```python
from build123d import *

# Parameters (mm, degrees)
SKETCH1_W           = 92
SKETCH1_H           = 56
BOSS_EXTRUDE1_DEPTH = 12
SKETCH8_W           = 92
SKETCH8_H           = 2
BOSS_EXTRUDE3_DEPTH = 12
CUT_EXTRUDE1_REACH  = 58.214
SKETCH2_R           = 10.5
CUT_EXTRUDE5_REACH  = 58.214
FILLET2_R           = 12
CUT_EXTRUDE6_DEPTH  = 6
CUT_EXTRUDE7_REACH  = 58.214
SKETCH12_R          = 2.25
SKETCH12_R_2        = 10.5


with BuildPart() as part:
    # Sketch1 → Boss-Extrude1 (new body)
    with BuildSketch(Plane(origin=(0, 0, 0), x_dir=(1, 0, 0), z_dir=(0, 1, 0))):
        Rectangle(SKETCH1_W, SKETCH1_H)
    extrude(amount=BOSS_EXTRUDE1_DEPTH)

    # Sketch8 → Boss-Extrude3 (add)
    with BuildSketch(Plane(origin=(0, 12, 0), x_dir=(1, 0, 0), z_dir=(0, 1, 0))):
        with Locations((0, 29)):
            Rectangle(SKETCH8_W, SKETCH8_H)
    extrude(amount=-BOSS_EXTRUDE3_DEPTH)

    # Sketch2 → Cut-Extrude1 (cut, up to next)
    with BuildSketch(Plane(origin=(0, 12, 0), x_dir=(1, 0, 0), z_dir=(0, 1, 0)), mode=Mode.PRIVATE) as cut_extrude1_sk1:
        with Locations(Location((-25, -1.5, 0), (0, 0, 270))):
            Circle(SKETCH2_R)
    cut_extrude1_tool1 = extrude(cut_extrude1_sk1.sketch, amount=-CUT_EXTRUDE1_REACH, mode=Mode.PRIVATE) & part.part
    # Sketch2 → Cut-Extrude1 (cut, up to next)
    with BuildSketch(Plane(origin=(0, 12, 0), x_dir=(1, 0, 0), z_dir=(0, 1, 0)), mode=Mode.PRIVATE) as cut_extrude1_sk2:
        with Locations(Location((25, -1.5, 0), (0, 0, 270))):
            Circle(SKETCH2_R)
    cut_extrude1_tool2 = extrude(cut_extrude1_sk2.sketch, amount=-CUT_EXTRUDE1_REACH, mode=Mode.PRIVATE) & part.part
    add(cut_extrude1_tool1.solids().sort_by_distance((-25, 12, 1.5))[0], mode=Mode.SUBTRACT)
    add(cut_extrude1_tool2.solids().sort_by_distance((25, 12, 1.5))[0], mode=Mode.SUBTRACT)

    # Sketch10 → Cut-Extrude5 (cut, up to next)
    with BuildSketch(Plane(origin=(0, 12, 0), x_dir=(1, 0, 0), z_dir=(0, 1, 0)), mode=Mode.PRIVATE) as cut_extrude5_sk1:
        with BuildLine():
            Line((-46, 5.057438524), (-46, 30))
            Line((-46, 30), (-16, 30))
            Line((-16, 30), (-35.667304108, 17.740806196))
            ThreePointArc((-35.667304108, 17.740806196), (-42.056420822, 12.395269294), (-46, 5.057438524))
        make_face()
    cut_extrude5_tool1 = extrude(cut_extrude5_sk1.sketch, amount=-CUT_EXTRUDE5_REACH, mode=Mode.PRIVATE) & part.part
    # Sketch10 → Cut-Extrude5 (cut, up to next)
    with BuildSketch(Plane(origin=(0, 12, 0), x_dir=(1, 0, 0), z_dir=(0, 1, 0)), mode=Mode.PRIVATE) as cut_extrude5_sk2:
        with BuildLine():
            Line((46, 5.057438524), (46, 30))
            Line((46, 30), (16, 30))
            Line((16, 30), (36.615382461, 17.183760068))
            ThreePointArc((36.615382461, 17.183760068), (42.39835371, 11.964668142), (46, 5.057438524))
        make_face()
    cut_extrude5_tool2 = extrude(cut_extrude5_sk2.sketch, amount=-CUT_EXTRUDE5_REACH, mode=Mode.PRIVATE) & part.part
    add(cut_extrude5_tool1.solids().sort_by_distance((-36.403407, 12, -23.114901))[0], mode=Mode.SUBTRACT)
    add(cut_extrude5_tool2.solids().sort_by_distance((36.411287, 12, -23.11647))[0], mode=Mode.SUBTRACT)

    # Fillet2
    fillet2_edges = [part.edges().sort_by_distance(p)[0] for p in [
        (-16, 6, -30),
        (16, 6, -30),
    ]]
    fillet(fillet2_edges, radius=FILLET2_R)

    # Sketch11 → Cut-Extrude6 (cut)
    with BuildSketch(Plane.XZ):
        with BuildLine():
            Line((22, -16.5), (22, -26.269899929))
            Line((22, -26.269899929), (16.545392108, -31))
            Line((16.545392108, -31), (-16.545392108, -31))
            Line((-16.545392108, -31), (-22, -26.260028196))
            Line((-22, -26.260028196), (-22, -16.5))
            ThreePointArc((-22, -16.5), (-20.591243605, -8.753988974), (-16.545392108, -2))
            Line((-16.545392108, -2), (16.545392108, -2))
            ThreePointArc((16.545392108, -2), (20.591243605, -8.753988974), (22, -16.5))
        make_face()
    extrude(amount=-CUT_EXTRUDE6_DEPTH, mode=Mode.SUBTRACT)

    # Sketch12 → Cut-Extrude7 (cut, up to next)
    with BuildSketch(Plane.XZ, mode=Mode.PRIVATE) as cut_extrude7_sk1:
        with Locations(Location((16, -16.5, 0), (0, 0, 270))):
            Circle(SKETCH12_R)
    cut_extrude7_tool1 = extrude(cut_extrude7_sk1.sketch, amount=-CUT_EXTRUDE7_REACH, mode=Mode.PRIVATE) & part.part
    # Sketch12 → Cut-Extrude7 (cut, up to next)
    with BuildSketch(Plane.XZ, mode=Mode.PRIVATE) as cut_extrude7_sk2:
        with Locations(Location((-16, -16.5, 0), (0, 0, 270))):
            Circle(SKETCH12_R)
    cut_extrude7_tool2 = extrude(cut_extrude7_sk2.sketch, amount=-CUT_EXTRUDE7_REACH, mode=Mode.PRIVATE) & part.part
    # Sketch12 → Cut-Extrude7 (cut, up to next)
    with BuildSketch(Plane.XZ, mode=Mode.PRIVATE) as cut_extrude7_sk3:
        with Locations(Location((0, -16.5, 0), (0, 0, 270))):
            Circle(SKETCH12_R_2)
    cut_extrude7_tool3 = extrude(cut_extrude7_sk3.sketch, amount=-CUT_EXTRUDE7_REACH, mode=Mode.PRIVATE) & part.part
    add(cut_extrude7_tool1.solids().sort_by_distance((16, 0, -16.5))[0], mode=Mode.SUBTRACT)
    add(cut_extrude7_tool2.solids().sort_by_distance((-16, 0, -16.5))[0], mode=Mode.SUBTRACT)
    add(cut_extrude7_tool3.solids().sort_by_distance((0, 0, -16.5))[0], mode=Mode.SUBTRACT)


solid = part.part
```
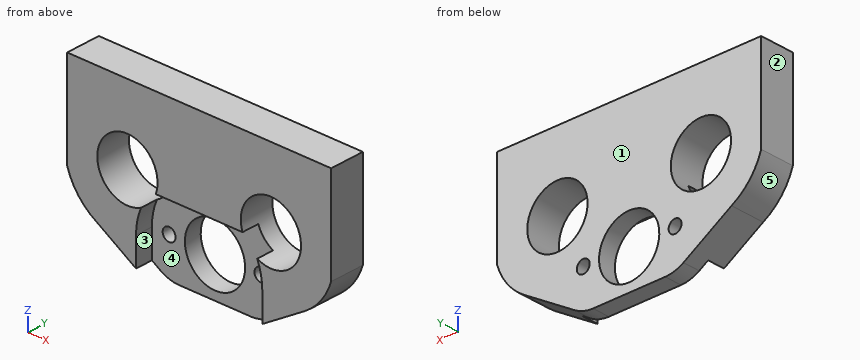
Work out the finished part from the listing and answer in its coordinate system (mm). Face numbers are marked on the shaded views. A direction names the side the tool comes from. Round coordinates to 2 decimals unless told otherwise and drop trailing zeros. Loops run counter-clockwise (first coordinate to the right, second up) from the corner with the lowest first, then second, coordinate; pieces in that order, holes last.
(1) The part is cut by section C-C, the plane y = 7.75. Give the vertices of the cut face in (x, z).
Computed values:
outline: (-46, -5.06) arc R22 ccw to (-35.67, -17.74) - (-18.91, -28.18) arc R12 ccw to (-12.57, -30) - (12.57, -30) arc R12 ccw to (18.91, -28.19) - (36.62, -17.18) arc R22 ccw to (46, -5.06) - (46, 28) - (-46, 28) - close; hole circle Ø21 at (-25, 1.5); hole circle Ø4.5 at (-16, -16.5); hole circle Ø21 at (0, -16.5); hole circle Ø4.5 at (16, -16.5); hole circle Ø21 at (25, 1.5)
(2) Find the intervals of material crossed by L1, parallel to X at y = 9.25, z = 1.5; L2, parallel to X at y = 9.5, z = -0.5; L3, parallel to X at y = 10.7, z = -16.5, in increasing order.
Computed values:
L1: x = -46 to -35.5, -14.5 to 14.5, 35.5 to 46
L2: x = -46 to -35.31, -14.69 to 14.69, 35.31 to 46
L3: x = -37.65 to -18.25, -13.75 to -10.5, 10.5 to 13.75, 18.25 to 37.65
(3) Each of these flat-tipped pins is pushed along its axis until it touches: P1, Ø1.8, axis at x = 5.5, y = 3, coming from the -Z side; P2, Ø1.5, axis at y = 7.5, z = -14, coming from the -X side; P3, Ø6, axis at x = 16, z = -16.5, coming from the -Y side. Where does it stop, or does it pass through?
Computed values:
P1: stops at z = -2
P2: stops at x = -41.32
P3: stops at y = 6
(4) The part is cut by section D-D, the plane x = -16. Give the vertices of the cut face in (y, z), and give its area (3 significant figures).
Computed values:
outline: (0, 6.91) - (12, 6.91) - (12, 28) - (0, 28) - close; (6, -29.5) - (12, -29.5) - (12, -18.75) - (6, -18.75) - close; (6, -14.25) - (12, -14.25) - (12, -3.91) - (6, -3.91) - close
area: 380 mm2
(5) The part is cut by section B-B, the plane x = 0. Give the vertices of the cut face in (y, z), and give its area (3 significant figures).
Computed values:
outline: (0, -2) - (6, -2) - (6, -6) - (12, -6) - (12, 28) - (0, 28) - close; (6, -30) - (12, -30) - (12, -27) - (6, -27) - close
area: 402 mm2
(6) The part is cut by section A-A, the plane z = 1.5. Give the vertices of the cut face in (x, y).
Computed values:
outline: (-46, 0) - (-35.5, 0) - (-35.5, 12) - (-46, 12) - close; (-14.5, 0) - (14.5, 0) - (14.5, 12) - (-14.5, 12) - close; (35.5, 0) - (46, 0) - (46, 12) - (35.5, 12) - close
(7) For the marked faces 4 and 5, determine the directions among +Z, -Z, +X, -X, +Y, -Y from which every point of the face is accessible in a straight line to the end or side of a thin tool.
Computed values:
face 4: -Z, -Y
face 5: -Z, -X, +Y, -Y
(8) The mould has two halves that part along X. Classify the marked faces 1, 2 and 3: pulls with the +X half, pulls with the -X half, needs draft (parallel to the pull), parting line crosses it, or undercut.
Computed values:
face 1: needs draft
face 2: pulls with the -X half
face 3: undercut
